Geometry: final body of the model. Coordinates: model frame, mm. A direction names the side the tool comes from. Give positions to 0.01 mm unless a question says otherwise; leave off trailing zeros. Order: outer loops, then holes, each group sorted by start corner. A loop starts at its lowest first (then second) coordinate and runs counter-clockwise, first axis right, second up. Notation, with made-up numbers: (25, 3.5) - (79, 3.5) arc R32 ccw to (79, 29.5) - close; hole circle Ø9 at (19.25, 56.25). An arc over 180 degrees is marked (long way). Put each result on its own line as item: value. Start each with the question number.
1. Set-up query: faces 5 (the flat face through (102.6, -24.5, 3)), 6 (the flat face through (58, 5, -10)), 7 (the flat face through (14.78, -19.73, 2.96)). Return all of +Z, -Z, +X, -X, +Y, -Y with unobstructed straight access to the full face (end or side cutting, diameter ignored); none if empty.
2. Mould query, pull axis X, two halves, no side actions, for faces 1 (the flat face through (8.62, -21.52, 2.96)), 2 (the flat face through (108.48, -21.65, 2.96)), 3 (the flat face through (14.6, -24.5, 3)), 4 (the flat face through (58, -12, 0)). Classes: pulls with the +X half, pulls with the -X half, needs draft (parallel to the pull), parting line crosses it, or undercut.
3. Section B-B on x = 58.6. Return the cut outline in (y, z).
4. First-contact query: P1, Ø6, axis at x = 94.5, z = -2, coming from the -Y side; P2, Ø3.5, axis at x = 74.1, y = -39.4, coming from the -Z side; P3, Ø8, axis at y = -17, z = -0.5, coming from the -X side. Flat tips, straight axial feed; report the tip coordinate or a pass-through.
5. Ray query, line 1 along X through (y, z) = (-9, 2.75); line 2 along Y through (x, z) = (74.6, 3.4); line 3 along Y through (x, z) = (43.1, 3.4). Return the intervals inside material, ascending. Write a range as from..to.
6. Section C-C on y = 9. Return the cut outline in (x, z), plus the area to 3 significant figures.
7. Section D-D on x = 34. Return the cut outline in (y, z).
8. Section A-A on z = 1.25. Count the separate pieces of the cut face and the enclosed holes in it, plus the area to 3 significant figures.
from build123d import *

# Parameters (mm, degrees)
F0_R     = 1.1
F0_R_2   = 10
F0_R_3   = 1.65
F1_DEPTH = 6
F2_W     = 5
F2_H     = 20
F3_DEPTH = 117.2


with BuildPart() as f1:
    # F0 (on Top) → F1 (new body)
    with BuildSketch(Plane.XY):
        with BuildLine():
            Line((0, 25), (0, 0))
            Line((0, 0), (0, -9))
            ThreePointArc((0, -9), (8.6, -0.4), (17.2, -9))
            ThreePointArc((17.2, -9), (16.5999275153, -12.1561305026), (14.8834512211, -14.8718174999))
            Line((14.8834512211, -14.8718174999), (37.5, -45))
            Line((37.5, -45), (79.7, -45))
            Line((79.7, -45), (102.3165487789, -14.8718174999))
            ThreePointArc((102.3165487789, -14.8718174999), (105.4438694974, -1.0000724847), (117.2, -9))
            Line((117.2, -9), (117.2, 25))
            Line((117.2, 25), (0, 25))
        make_face()
        with Locations((43.1, -39.4)):
            Circle(F0_R, mode=Mode.SUBTRACT)
        with Locations((74.1, -39.4)):
            Circle(F0_R, mode=Mode.SUBTRACT)
        with Locations((58.6, -23.9)):
            Circle(F0_R_2, mode=Mode.SUBTRACT)
        with Locations((43.1, -8.4)):
            Circle(F0_R, mode=Mode.SUBTRACT)
        with Locations((24.6, 15)):
            Circle(F0_R_3, mode=Mode.SUBTRACT)
        with Locations((42.6, 15)):
            Circle(F0_R_3, mode=Mode.SUBTRACT)
        with Locations((74.1, -8.4)):
            Circle(F0_R, mode=Mode.SUBTRACT)
        with Locations((74.6, 15)):
            Circle(F0_R_3, mode=Mode.SUBTRACT)
        with Locations((92.6, 15)):
            Circle(F0_R_3, mode=Mode.SUBTRACT)
        with BuildLine():
            ThreePointArc((17.2, -9), (8.6, -0.4), (0, -9))
            ThreePointArc((0, -9), (1.3952892231, -13.6959708922), (5.1284052606, -16.8681656036))
            ThreePointArc((5.1284052606, -16.8681656036), (8.8282621536, -17.5969701866), (12.484231675, -16.6728576355))
            Line((12.484231675, -16.6728576355), (9.6911672785, -12.9521328381))
            ThreePointArc((9.6911672785, -12.9521328381), (5.3378085708, -6.5164325902), (12.7, -9))
            ThreePointArc((12.7, -9), (12.5446537225, -10.1179029518), (12.0903868245, -11.1510927026))
            Line((12.0903868245, -11.1510927026), (14.8834512211, -14.8718174999))
            ThreePointArc((14.8834512211, -14.8718174999), (16.5999275153, -12.1561305026), (17.2, -9))
        make_face()
        with BuildLine():
            ThreePointArc((12.484231675, -16.6728576355), (8.8282621536, -17.5969701866), (5.1284052606, -16.8681656036))
            Line((5.1284052606, -16.8681656036), (12.2074985246, -26.2984379178))
            Line((12.2074985246, -26.2984379178), (17.0059376167, -22.6963576466))
            Line((17.0059376167, -22.6963576466), (12.484231675, -16.6728576355))
        make_face()
        with BuildLine():
            ThreePointArc((112.0715947394, -16.8681656036), (115.8047107769, -13.6959708922), (117.2, -9))
            ThreePointArc((117.2, -9), (105.4438694974, -1.0000724847), (102.3165487789, -14.8718174999))
            Line((102.3165487789, -14.8718174999), (105.1096131755, -11.1510927026))
            ThreePointArc((105.1096131755, -11.1510927026), (107.4820970482, -5.0553462775), (112.7, -9))
            ThreePointArc((112.7, -9), (111.0835674098, -12.2621914292), (107.5088327215, -12.9521328381))
            Line((107.5088327215, -12.9521328381), (104.715768325, -16.6728576355))
            ThreePointArc((104.715768325, -16.6728576355), (108.3717378464, -17.5969701866), (112.0715947394, -16.8681656036))
        make_face()
        with BuildLine():
            ThreePointArc((12.484231675, -16.6728576355), (13.762981722, -15.8777626986), (14.8834512211, -14.8718174999))
            Line((14.8834512211, -14.8718174999), (12.0903868245, -11.1510927026))
            ThreePointArc((12.0903868245, -11.1510927026), (11.0614215186, -12.2789333796), (9.6911672785, -12.9521328381))
            Line((9.6911672785, -12.9521328381), (12.484231675, -16.6728576355))
        make_face()
        with BuildLine():
            Line((105.1096131755, -11.1510927026), (102.3165487789, -14.8718174999))
            ThreePointArc((102.3165487789, -14.8718174999), (103.437018278, -15.8777626986), (104.715768325, -16.6728576355))
            Line((104.715768325, -16.6728576355), (107.5088327215, -12.9521328381))
            ThreePointArc((107.5088327215, -12.9521328381), (106.1385784814, -12.2789333796), (105.1096131755, -11.1510927026))
        make_face()
        with BuildLine():
            Line((104.9925014754, -26.2984379178), (112.0715947394, -16.8681656036))
            ThreePointArc((112.0715947394, -16.8681656036), (108.3717378464, -17.5969701866), (104.715768325, -16.6728576355))
            Line((104.715768325, -16.6728576355), (100.1940623833, -22.6963576466))
            Line((100.1940623833, -22.6963576466), (104.9925014754, -26.2984379178))
        make_face()
    extrude(amount=F1_DEPTH)

    # F2 (on Right) → F3 (join)
    with BuildSketch(Plane.YZ):
        with Locations((2.5, -10)):
            Rectangle(F2_W, F2_H)
    extrude(amount=F3_DEPTH)


solid = f1.part
Resolved:
1. face 5: +Z, -Z, -Y
1. face 6: -Z, +X, -X, +Y
1. face 7: +Z, -Z
2. face 1: pulls with the -X half
2. face 2: pulls with the +X half
2. face 3: undercut
2. face 4: needs draft
3. outline: (-45, 0) - (-33.9, 0) - (-33.9, 6) - (-45, 6) - close; (-13.9, 0) - (0, 0) - (0, -20) - (5, -20) - (5, 0) - (25, 0) - (25, 6) - (-13.9, 6) - close
4. P1: y = -28.26
4. P2: z = 0
4. P3: x = 1
5. line 1: 0..4.5, 12.7..42.18, 44.02..73.18, 75.02..104.5, 112.7..117.2
5. line 2: -45..-40.38, -38.42..-9.38, -7.42..13.35, 16.65..25
5. line 3: -45..-40.5, -38.3..-9.5, -7.3..13.43, 16.57..25
6. outline: (0, 0) - (117.2, 0) - (117.2, 6) - (0, 6) - close
6. area: 703 mm^2
7. outline: (-40.34, 0) - (0, 0) - (0, -20) - (5, -20) - (5, 0) - (25, 0) - (25, 6) - (-40.34, 6) - close
8. separate pieces: 1
8. enclosed holes: 11
8. area: 6,300 mm^2
